from build123d import *

# Parameters (mm, degrees)
SKETCH1_W               = 412
SKETCH1_H               = 515
BASE_FLANGE1_DEPTH      = 1
EDGE_FLANGE1_DEPTH      = 412
EDGE_FLANGE2_DEPTH      = 412
CUT_EXTRUDE1_DEPTH      = 349.464130148
CUT_EXTRUDE1_DEPTH_BACK = 349.464130148
SKETCH12_R              = 3.05


# Sheet-metal steps are written as plain solids
with BuildPart() as part:
    # Sketch1 → Base-Flange1 (new body)
    with BuildSketch(Plane(origin=(0, 0, 0), x_dir=(1, 0, 0), z_dir=(0, 1, 0))):
        Rectangle(SKETCH1_W, SKETCH1_H)
    extrude(amount=-BASE_FLANGE1_DEPTH)

    # Edge-Flange1 section (across the edge) → Edge-Flange1 (add)
    with BuildSketch(Plane(origin=(-206, -1, -260.5), x_dir=(0, 0, 1), z_dir=(1, 0, 0))):
        with BuildLine():
            Line((-1, 3), (-1, 98))
            Line((-1, 98), (0, 98))
            Line((0, 98), (0, 3))
            ThreePointArc((0, 3), (0.878679656, 0.878679656), (3, 0))
            Line((3, 0), (3, -1))
            ThreePointArc((3, -1), (0.171572875, 0.171572875), (-1, 3))
        make_face()
    extrude(amount=EDGE_FLANGE1_DEPTH)

    # Edge-Flange2 section (across the edge) → Edge-Flange2 (add)
    with BuildSketch(Plane(origin=(-206, -102, -260.5), x_dir=(0, 1, 0), z_dir=(1, 0, 0))):
        with BuildLine():
            Line((-1, 3), (-1, 449))
            Line((-1, 449), (0, 449))
            Line((0, 449), (0, 3))
            ThreePointArc((0, 3), (0.878679656, 0.878679656), (3, 0))
            Line((3, 0), (3, -1))
            ThreePointArc((3, -1), (0.171572875, 0.171572875), (-1, 3))
        make_face()
    extrude(amount=EDGE_FLANGE2_DEPTH)

    # Sketch12 → Cut-Extrude1 (cut, two sides: drawn at the far end of the back side and taken through both)
    with BuildSketch(Plane(origin=(0, 0, 0), x_dir=(1, 0, 0), z_dir=(0, 1, 0)).offset(-CUT_EXTRUDE1_DEPTH_BACK)):
        with Locations(Location((196, 177.5, 0), (0, 0, 270))):
            Circle(SKETCH12_R)
        with Locations(Location((196, 94.45, 0), (0, 0, 270))):
            Circle(SKETCH12_R)
        with Locations(Location((196, 11.4, 0), (0, 0, 270))):
            Circle(SKETCH12_R)
        with Locations(Location((196, -71.65, 0), (0, 0, 270))):
            Circle(SKETCH12_R)
        with Locations(Location((196, -154.7, 0), (0, 0, 270))):
            Circle(SKETCH12_R)
        with Locations(Location((196, -237.75, 0), (0, 0, 90))):
            Circle(SKETCH12_R)
        with Locations(Location((-196, -237.75, 0), (0, 0, 90))):
            Circle(SKETCH12_R)
        with Locations(Location((-196, -154.7, 0), (0, 0, 270))):
            Circle(SKETCH12_R)
        with Locations(Location((-196, -71.65, 0), (0, 0, 270))):
            Circle(SKETCH12_R)
        with Locations(Location((-196, 11.4, 0), (0, 0, 270))):
            Circle(SKETCH12_R)
        with Locations(Location((-196, 94.45, 0), (0, 0, 270))):
            Circle(SKETCH12_R)
        with Locations(Location((-196, 177.5, 0), (0, 0, 270))):
            Circle(SKETCH12_R)
    extrude(amount=CUT_EXTRUDE1_DEPTH + CUT_EXTRUDE1_DEPTH_BACK, mode=Mode.SUBTRACT)


solid = part.part
The listing builds one solid part. Answer for the finished solid, in the listing's coordinates (mm). A direction names the side the tool comes from. Coordinates: 2 decimals unless noted, no trailing zeros. Write each loop counter-clockwise with the first axis right and the second up, starting at its lowest first coordinate (ties: lowest second). Pieces come first, ordered by that corner, then holes. Notation, with made-up numbers: (33, -7) - (53, -7) arc R26 cw to (53, 23) - close; hole circle Ø5 at (70, 24.25). An arc over 180 degrees is marked (long way). Put each result on its own line as item: value.
1. The part is cut by section A-A on z = 61. Give the vertices of the cut face in (x, y).
Answer sheet:
outline: (-206, -103) - (206, -103) - (206, -102) - (-206, -102) - close; (-206, -1) - (206, -1) - (206, 0) - (-206, 0) - close
2. Determine the mould class of faces 3 (the face through (-3, 0, -4)), 4 (the face through (-3, -51, -261.5)), 5 (the face through (-3, -1, -4)) for opening direction Y: pulls with the +Y half, pulls with the -Y half, needs draft (parallel to the pull), parting line crosses it, or undercut.
Answer sheet:
face 3: pulls with the +Y half
face 4: needs draft
face 5: undercut
3. Flat-ended cylindrical pins translate along their axes: pin 1 Ø10 at (x, z) = (196, 71.65) entering from +Y; pin 2 Ø2 at (x, y) = (-98.5, -71) entering from +Z. Find the tip coordinate at first contact, or state that the pin passes through.
Answer sheet:
pin 1: stops at y = 0
pin 2: stops at z = -260.5
4. The part is cut by section B-B on x = 177.5. Give the vertices of the cut face in (y, z), plus the area to 3 significant figures.
Answer sheet:
outline: (-103, -257.5) arc R4 ccw to (-99, -261.5) - (-4, -261.5) arc R4 ccw to (0, -257.5) - (0, 257.5) - (-1, 257.5) - (-1, -257.5) arc R3 cw to (-4, -260.5) - (-99, -260.5) arc R3 cw to (-102, -257.5) - (-102, 188.5) - (-103, 188.5) - close
area: 1,070 mm^2
5. The part is cut by section C-C on y = -39. Give the vertices of the cut face in (x, z).
Answer sheet:
outline: (-206, -261.5) - (206, -261.5) - (206, -260.5) - (-206, -260.5) - close
6. Find the intervals of material crossed by line 1 along X through (y, z) = (-0.25, -177.5); line 2 along Y through (x, z) = (-139, 169); line 3 along Y through (x, z) = (-46, 202), in increasing order. Write a range as from..to.
Answer sheet:
line 1: x = -206..-199.05, -192.95..192.95, 199.05..206
line 2: y = -103..-102, -1..0
line 3: y = -1..0
7. A tool of negligible diameter and unlimited length cuts with its end or side. For faces 1 (the face through (-3, -103, -38)), 2 (the face through (-3, -52, -260.5)), from which of +Z, -Z, +X, -X, +Y, -Y can it reach the whole face along a straight path? Write none if from no direction.
Answer sheet:
face 1: +Z, -Z, +X, -X, -Y
face 2: +Z, +X, -X
